Part model, mm, in its own coordinate system. A direction names the side the tool comes from. Coordinates: 2 decimals unless noted, no trailing zeros. Order: outer loops, then holes, each group sorted by start corner. A loop starts at its lowest first (then second) coordinate and runs counter-clockwise, first axis right, second up.
from build123d import *

# Parameters (mm, degrees)
CUT_EXTRUDE2_DEPTH = 3


with BuildPart() as part:
    # Sketch3 → Revolve2 (revolve)
    with BuildSketch(Plane.XY):
        Polygon((0, 0), (-5, 0), (-5, -4), (-3, -4), (-3, -44), (-2.5, -44), (-2.5, -54), (0, -54), align=None)
    revolve(axis=Axis((0, 0, 0), (0, -1, 0)))

    # Sketch4 → Cut-Extrude2 (cut)
    with BuildSketch(Plane(origin=(0, 0, 0), x_dir=(1, 0, 0), z_dir=(0, 1, 0))):
        Polygon((1.5, 0.866025404), (0, 1.732050808), (-1.5, 0.866025404), (-1.5, -0.866025404), (0, -1.732050808), (1.5, -0.866025404), align=None)
    extrude(amount=-CUT_EXTRUDE2_DEPTH, mode=Mode.SUBTRACT)


solid = part.part
Q1. Cut at D-D on x = -4.25. Write the cut outline in (y, z), and give its area (3 significant figures).
Results list:
outline: (-4, -2.63) - (0, -2.63) - (0, 2.63) - (-4, 2.63) - close
area: 21.1 mm2
Q2. Which spindle directions (+Z, -Z, +X, -X, +Y, -Y) get a long thin tool onto all of the face, cutting with end or side? Do faces 1 (the face through (0.54, -49.07, 2.44)), 2 (the face through (1.5, -1, 0)), 3 (the face through (2, 0, 0)). Say none if no direction does.
Results list:
face 1: -Y
face 2: +Y
face 3: +Z, -Z, +X, -X, +Y
Q3. Cut at C-C on x = 4. Write the cut outline in (y, z).
Results list:
outline: (-4, -3) - (0, -3) - (0, 3) - (-4, 3) - close
Q4. Cut at B-B on y = -16. Write the cut outline in (x, z), and give its area (3 significant figures).
Results list:
outline: circle Ø6 at (0, 0)
area: 28.3 mm2
Q5. Mould opens along X. For faces 4 (the face through (1.08, -2.03, 4.88)), 5 (the face through (0.76, -1.479, -1.293)), 6 (the face through (2, -44, -2)) say: pulls with the +X half, pulls with the -X half, needs draft (parallel to the pull), parting line crosses it, or undercut.
Results list:
face 4: parting line crosses it
face 5: undercut
face 6: needs draft
Q6. Wall check: line 1 along Z through (x, y) = (0.25, -43); line 2 along Y through (x, z) = (2.5, -4); line 3 along Y through (x, z) = (-2.5, -1). Give the ranges that are in metal, low to high.
Results list:
line 1: z = -2.99 to 2.99
line 2: y = -4 to 0
line 3: y = -44 to 0
Q7. Pin check, flat tips, straight feed: pin 1 Ø1 at (x, y) = (0.5, -30.5) entering from -Z; pin 2 Ø6 at (y, z) = (-13.5, 0) entering from -X; pin 3 Ø3 at (x, y) = (-3, -16) entering from +Z. Stop position of each tip, or through.
Results list:
pin 1: stops at z = -3
pin 2: stops at x = -3
pin 3: stops at z = 2.6
Q8. Cut at A-A on z = 0. Write the cut outline in (x, y).
Results list:
outline: (-5, -4) - (-3, -4) - (-3, -44) - (-2.5, -44) - (-2.5, -54) - (2.5, -54) - (2.5, -44) - (3, -44) - (3, -4) - (5, -4) - (5, 0) - (1.5, 0) - (1.5, -3) - (-1.5, -3) - (-1.5, 0) - (-5, 0) - close
